Source: CAD feature listing. Evaluate the final solid. Frame: model axes, mm. Give positions to 0.01 mm unless a question says otherwise; leave off trailing zeros. Order: outer loops, then holes, each group sorted by start corner. A loop starts at its lowest first (then second) coordinate and runs counter-clockwise, first axis right, second up. Notation, with made-up numbers: (1, 51.25) -> (18, 51.25) arc R31 ccw to (18, 83.25) -> close; hole circle Ø5 at (89.5, 54.25). An arc over 180 degrees is marked (long way). Use CSV: the item, a comma, the result in double quotes.
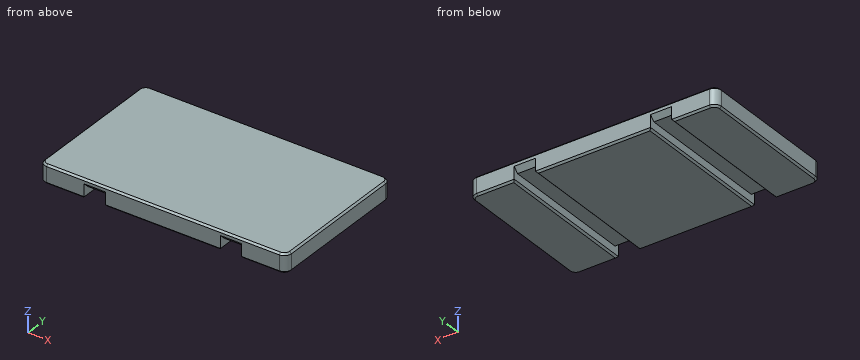
Autodesk Inventor part; units mm, degrees
ref_plane "YZ Plane" through (0, 0, 0) normal (1, 0, 0) x (0, 1, 0)
ref_plane "XZ Plane" through (0, 0, 0) normal (0, 1, 0) x (-1, 0, 0)
ref_plane "XY Plane" through (0, 0, 0) normal (0, 0, 1) x (1, 0, 0)
sketch "Sketch1" plane through (0, 0, 0) normal (0, 0, 1) x (1, 0, 0)
  line L0 (-52.5, -31) -> (52.5, -31)
  line L1 (52.5, -31) -> (52.5, 31)
  line L2 (52.5, 31) -> (-52.5, 31)
  line L3 (-52.5, 31) -> (-52.5, -31)
  line L4 (-52.5, -31) -> (52.5, 31) construction
  line L5 (52.5, -31) -> (-52.5, 31) construction
  point P0 (0, 0)
  dimension "d1" = 105
  dimension "d2" = 62
extrude "Extrusion1" add sketch "Sketch1" along normal blind 8
sketch "Sketch2" plane through (0, 0, 0) normal (0, 0, -1) x (-1, 0, 0)
  line L0 (-52.5, -31) -> (-52.5, 31)
  line L1 (52.5, -31) -> (-52.5, -31)
  line L2 (52.5, 31) -> (52.5, -31)
  line L3 (-52.5, 31) -> (52.5, 31)
  line L4 (52.5, -31) -> (-52.5, -31)
  line L5 (33.5, -31) -> (24.5, -31)
  line L6 (24.5, -31) -> (24.5, 31)
  line L7 (24.5, 31) -> (33.5, 31)
  line L8 (33.5, 31) -> (33.5, -31)
  line L9 (-73.5, 0) -> (73.5, 0) construction
  line L10 (0, -43.4) -> (0, 43.4) construction
  line L11 (-33.5, -31) -> (-24.5, -31)
  line L12 (-24.5, -31) -> (-24.5, 31)
  line L13 (-24.5, 31) -> (-33.5, 31)
  line L14 (-33.5, 31) -> (-33.5, -31)
  point P0 (0, 0)
  point P1 (-33.5, 31)
  point P2 (-24.5, 31)
  point P3 (33.5, 31)
  dimension "d5" = 9
  dimension "d6" = 19
extrude "Extrusion2" cut sketch "Sketch2" against normal blind 4 contours L14 L3 L12 L1 | L6 L3 L8 L1
chamfer "Chamfer1" distance 2 angle 45 4 edges at (-29, -31, 4) (29, -31, 4) (29, 31, 4) (-29, 31, 4)
fillet "Fillet1" radius 3 4 edges at (-52.5, -31, 4) (-52.5, 31, 4) (52.5, -31, 4) (52.5, 31, 4)
chamfer "Chamfer2" distance 0.75 angle 45 4 edges at (0, -31, 8) (-52.5, 0, 8) (0, 31, 8) (52.5, 0, 8)
chamfer "Chamfer3" distance 0.75 angle 45 16 edges at (-52.5, 0, 0) (-51.6213, -30.1213, 0) (-41.5, -31, 0) (-51.6213, 30.1213, 0) (-41.5, 31, 0) (52.5, 0, 0) (51.6213, 30.1213, 0) (41.5, 31, 0) (51.6213, -30.1213, 0) (41.5, -31, 0) (0, 31, 0) (24.5, 0, 0) (0, -31, 0) (-24.5, 0, 0) (-33.5, 0, 0) (33.5, 0, 0)
properties part number "BatteryHolder_3DPrint"
1. Ray query, line 1 along X through (y, z) = (20.5, 0.75); line 2 along Z through (x, y) = (29.5, 21); line 3 along Y through (x, z) = (18.5, 7.5). Return the intervals inside material, ascending.
Answer below:
line 1,"x = -52.5 to -33.5, -24.5 to 24.5, 33.5 to 52.5"
line 2,"z = 4 to 8"
line 3,"y = -30.75 to 30.75"
2. Section query B-B on x = -28. Return loops of the section in (y, z).
Answer below:
outline,"(-31, 6) -> (-29, 4) -> (29, 4) -> (31, 6) -> (31, 7.25) -> (30.25, 8) -> (-30.25, 8) -> (-31, 7.25) -> close"
3. Section query C-C on y = -25.5. Return loops of the section in (x, z), plus the area to 3 significant figures.
Answer below:
outline,"(-52.5, 0.75) -> (-51.75, 0) -> (-34.25, 0) -> (-33.5, 0.75) -> (-33.5, 4) -> (-24.5, 4) -> (-24.5, 0.75) -> (-23.75, 0) -> (23.75, 0) -> (24.5, 0.75) -> (24.5, 4) -> (33.5, 4) -> (33.5, 0.75) -> (34.25, 0) -> (51.75, 0) -> (52.5, 0.75) -> (52.5, 7.25) -> (51.75, 8) -> (-51.75, 8) -> (-52.5, 7.25) -> close"
area,"766 mm²"
4. Section query A-A on z = 2. Return loops of the section in (x, y).
Answer below:
outline,"(-52.5, -28) arc R3 ccw to (-49.5, -31) -> (-33.5, -31) -> (-33.5, 31) -> (-49.5, 31) arc R3 ccw to (-52.5, 28) -> close; (-24.5, -31) -> (24.5, -31) -> (24.5, 31) -> (-24.5, 31) -> close; (33.5, -31) -> (49.5, -31) arc R3 ccw to (52.5, -28) -> (52.5, 28) arc R3 ccw to (49.5, 31) -> (33.5, 31) -> close"
5. Pin query (flat end, axial travel): P1, Ø2.5, axis at x = 31, y = 5, coming from the -Z side. Return the tip coordinate at first contact, or that it passes through.
Answer below:
P1,"stops at z = 4"
